Geometry: final body of the model. Coordinates: model frame, mm. A direction names the side the tool comes from. Coordinates: 2 decimals unless noted, no trailing zeros. Order: outer loops, then holes, each group sorted by start corner. A loop starts at its lowest first (then second) coordinate and runs counter-clockwise, first axis right, second up. Notation, with made-up numbers: M -20.75,9 L 38.25,9 A13 cw 38.25,31 Z; hole C 27,59.5 d1. An arc over 180 degrees is marked long. One line per question, with ' | ' between items.
from build123d import *

# Parameters (mm, degrees)
SKETCH1_W           = 19
SKETCH1_H           = 19
BOSS_EXTRUDE1_DEPTH = 6
SKETCH2_R           = 4.5
BOSS_EXTRUDE2_DEPTH = 76
SKETCH13_OUTSIDE_W  = 59.042
SKETCH13_OUTSIDE_H  = 59.042
SKETCH13_OUTSIDE_R  = 9.5
CUT_EXTRUDE1_DEPTH  = 6
CUT_EXTRUDE1_DRAFT  = -60


with BuildPart() as part:
    # Sketch1 → Boss-Extrude1 (new body)
    with BuildSketch(Plane(origin=(0, 0, 0), x_dir=(1, 0, 0), z_dir=(0, 1, 0))):
        with Locations((9.5, 9.5)):
            Rectangle(SKETCH1_W, SKETCH1_H)
    extrude(amount=BOSS_EXTRUDE1_DEPTH)

    # Sketch2 → Boss-Extrude2 (add)
    with BuildSketch(Plane(origin=(0, 6, 0), x_dir=(1, 0, 0), z_dir=(0, 1, 0))):
        with Locations(Location((9.5, 9.5, 0), (0, 0, 90))):  # turned: the seam where the file's is
            Circle(SKETCH2_R)
    extrude(amount=BOSS_EXTRUDE2_DEPTH)


with BuildPart() as cut_extrude1_tool:
    # Sketch13 outside → Cut-Extrude1 (with draft: the straight prism first)
    with BuildSketch(Plane(origin=(0, 0, 0), x_dir=(-1, 0, 0), z_dir=(0, -1, 0))):
        with Locations((-9.5, 9.5)):
            Rectangle(SKETCH13_OUTSIDE_W, SKETCH13_OUTSIDE_H)
        with Locations((-9.5, 9.5)):
            Circle(SKETCH13_OUTSIDE_R, mode=Mode.SUBTRACT)
    extrude(amount=-CUT_EXTRUDE1_DEPTH)
    # Cut-Extrude1: the draft: its side faces are tilted about the plane it starts from
    cut_extrude1_sides = [cut_extrude1_tool.faces().sort_by_distance(p)[0] for p in [
        (9.5, 3, 20.021),
        (-20.021, 3, -9.5),
        (9.5, 3, -39.021),
        (39.021, 3, -9.5),
        (19, 3, -9.5),
    ]]
    draft(cut_extrude1_sides, Plane(origin=(0, 0, 0), x_dir=(-1, 0, 0), z_dir=(0, -1, 0)), CUT_EXTRUDE1_DRAFT)


with BuildPart() as part_1:
    add(part.part)

    # Cut-Extrude1: cut by cut_extrude1_tool
    add(cut_extrude1_tool.part, mode=Mode.SUBTRACT)


solid = part_1.part
1. Material intervals for line 1 (Y direction, x = 2, z = -11); line 2 (X direction, y = 42, z = -9.75); line 3 (Y direction, x = 3.5, z = -2), sorted ascending. Write a range as [from, to].
Response values:
line 1: y = [0, 6] | line 2: x = [5.01, 13.99] | line 3: y = [0.06, 6]
2. Access query for faces 1 (the face through (9, 0, -10)), 2 (the face through (8.148, 43.468, -13.792)). Directions: +Z, -Z, +X, -X, +Y, -Y. A direction counts if a zero-diameter tool reaches every point of the face in a straight line with its end or side. Return the directions, or none.
Response values:
face 1: +Z, -Z, +X, -X, -Y | face 2: +Y
3. Pin query (flat end, axial travel): P1, Ø3, axis at x = 2.5, z = -3, coming from the -Y side; P2, Ø8, axis at y = 33.5, z = -3.5, coming from the +X side; P3, Ø10, axis at y = 51, z = -11, coming from the -X side; P4, Ø6, axis at y = 19, z = -3, coming from the +X side. Return the tip coordinate at first contact, or that it passes through.
Response values:
P1: stops at y = 0 | P2: stops at x = 13.53 | P3: stops at x = 5 | P4: stops at x = 12.33
4. Section A-A, the plane y = 69.5. Output: boundary loops of the cut face in (x, z), and give its area (3 significant figures).
Response values:
outline: C 9.5,-9.5 d9 | area: 63.6 mm^2
